from build123d import *

# Parameters (mm, degrees)
BOSS_EXTRUDE1_DEPTH  = 10
BOSS_EXTRUDE2_DEPTH  = 2.5
SKETCH9_W            = 14
SKETCH9_H            = 9
BOSS_EXTRUDE11_DEPTH = 4
SKETCH10_W           = 14
SKETCH10_H           = 8
BOSS_EXTRUDE12_DEPTH = 3


with BuildPart() as part:
    # Sketch1 → Boss-Extrude1 (new body)
    with BuildSketch(Plane.XY):
        Polygon((0, 1), (0, 0), (0, -9), (15.5, -9), (15.5, -5), (4, -5), (4, -0.5), (5.5, -0.5), (5.5, 1), align=None)
        Polygon((15.5, -5), (15.5, -9), (31, -9), (31, 0), (31, 1), (25.5, 1), (25.5, -0.5), (27, -0.5), (27, -5), align=None)
    extrude(amount=BOSS_EXTRUDE1_DEPTH)

    # Sketch2 → Boss-Extrude2 (add, symmetric)
    with BuildSketch(Plane.ZY.offset(-15.5)):
        Polygon((0, -9), (70.710678119, -79.710678119), (74.130879552, -70.313751911), (12.817127641, -9), align=None)
    extrude(amount=BOSS_EXTRUDE2_DEPTH, both=True)

    # Sketch9 → Boss-Extrude11 (add)
    with BuildSketch(Plane(origin=(0, -9, 0), x_dir=(1, 0, 0), z_dir=(0, 1, 0))):
        with Locations((15.5, -14.5)):
            Rectangle(SKETCH9_W, SKETCH9_H)
    extrude(amount=BOSS_EXTRUDE11_DEPTH)

    # Sketch10 → Boss-Extrude12 (add)
    with BuildSketch(Plane.XY.offset(19)):
        with Locations((15.5, -5)):
            Rectangle(SKETCH10_W, SKETCH10_H)
    extrude(amount=BOSS_EXTRUDE12_DEPTH)


solid = part.part
Work out the finished part from the listing and answer in its coordinate system (mm). A direction names the side the tool comes from. Coordinates: 2 decimals unless noted, no trailing zeros. Write each loop counter-clockwise with the first axis right and the second up, starting at its lowest first coordinate (ties: lowest second). Pieces come first, ordered by that corner, then holes. Notation, with made-up numbers: M 3,69 L 24,69 A18 cw 24,100 Z; hole C -11.5,17.25 d9. An arc over 180 degrees is marked long. Answer as CSV lines item,"result". Start each with the question number.
Item 1: Determine the mould class of faces 1 (the face through (15, -44, 35)), 2 (the face through (4, -3, 5)), 3 (the face through (27, -3, 5)), 4 (the face through (18, -42, 37)) for opening direction Y: released by +Y, released by -Y, zero draft, split by the parting line, or undercut.
Item 2: Section C-C on y = -74 is taken. Write down the section's boundary in (x, z).
Item 3: Section A-A on z = 14 is taken. Write down the section's boundary in (x, y).
Item 4: Consider L1, parallel to X at y = -42, z = 43.5; L2, parallel to Z at x = 25, y = -8.5; L3, parallel to Y at x = 10.5, z = 6. Determine where each line is inside the solid, lowest interval first.
Item 5: Section B-B on x = 15 is taken. Write down the section's boundary in (y, z), and give its area (3 significant figures).
Item 6: Flat-ended cylindrical pins translate along their axes: P1, Ø12, axis at x = 13, y = -70, coming from the +Z side; P2, Ø9, axis at x = 17.5, y = -4, coming from the +Z side; P3, Ø2.5, axis at x = 28, y = -4, coming from the +Z side; P4, Ø0.9, axis at x = 12.5, z = 21, coming from the +Y side. Find the tip coordinate at first contact, or state that the pin passes through.
Item 7: Section D-D on x = 28.5 is taken. Write down the section's boundary in (y, z), and give its area (3 significant figures).
Item 8: A tool of negligible diameter and unlimited length cuts with its end or side. For faces 5 (the face through (22.5, -6, 17)), 6 (the face through (15, -3, 19)), 7 (the face through (15, -5, 22)), from which of +Z, -Z, +X, -X, +Y, -Y can it reach the whole face along a straight path? Write none if from no direction.
Checks:
1,face 1,"released by -Y"
1,face 2,"undercut"
1,face 3,"undercut"
1,face 4,"zero draft"
2,outline,"M 13,65 L 18,65 L 18,72.79 L 13,72.79 Z"
3,outline,"M 8.5,-9 L 22.5,-9 L 22.5,-5 L 8.5,-5 Z; M 13,-23 L 18,-23 L 18,-10.18 L 13,-10.18 Z"
4,L1,"x = 13 to 18"
4,L2,"z = 0 to 10"
4,L3,"y = -9 to -5"
5,outline,"M -79.71,70.71 L -9,0 L -5,0 L -5,19 L -1,19 L -1,22 L -9,22 L -9,12.82 L -70.31,74.13 Z"
5,area,"946 mm²"
6,P1,"stops at z = 74.13"
6,P2,"stops at z = 22"
6,P3,"stops at z = 10"
6,P4,"stops at y = -1"
7,outline,"M -9,0 L 1,0 L 1,10 L -9,10 Z"
7,area,"100 mm²"
8,face 5,"+Z, +X, +Y, -Y"
8,face 6,"-Z, +X, -X, +Y"
8,face 7,"+Z, +X, -X, +Y"
